from build123d import *

# Parameters (mm, degrees)
F0_R     = 4
F1_DEPTH = 15
F2_R     = 2.4
F3_DEPTH = 8
F4_SIZE  = 0.8
F5_R     = 11
F6_DEPTH = 5


with BuildPart() as f1:
    # F0 (on Top) → F1 (new body)
    with BuildSketch(Plane.XY):
        Circle(F0_R)
    extrude(amount=F1_DEPTH)

    # F2 (on face) → F3 (join)
    with BuildSketch(Plane.XY.offset(15)):
        Circle(F2_R)
    extrude(amount=F3_DEPTH)

    # F4
    f4_edges = [f1.edges().sort_by_distance(p)[0] for p in [
        (-2.4, 0, 23),
        (-4, 0, 0),
    ]]
    chamfer(f4_edges, length=F4_SIZE)

    # F5 (on Right) → F6 (cut, symmetric)
    with BuildSketch(Plane.YZ):
        with Locations((-13.5, 8)):
            Circle(F5_R)
        with Locations((13.5, 8)):
            Circle(F5_R)
    extrude(amount=F6_DEPTH, both=True, mode=Mode.SUBTRACT)


solid = f1.part
Model file for the job. Use its own axes, mm. Give positions to 0.01 mm unless a question says otherwise; leave off trailing zeros. Order: outer loops, then holes, each group sorted by start corner. A loop starts at its lowest first (then second) coordinate and runs counter-clockwise, first axis right, second up. Notation, with made-up numbers: (84, -2.75) - (103, -2.75) arc R31 ccw to (103, 34.25) - close; hole circle Ø3 at (-28.5, -34). An arc over 180 degrees is marked (long way). Write item = value, one per line. Start each with the question number.
1. Cut at A-A, the plane y = 0. List the corners of the cut face in (x, z).
2. Drop flat-ended pins along their axis: P1, Ø1, axis at x = 1.5, y = -2, coming from the +Z side; P2, Ø1.5, axis at x = 2, z = 7, coming from the -Y side. Give the stop position or say it passes through.
3. Cut at D-D, the plane z = 11.25. List the corners of the cut face in (x, y).
4. Cut at B-B, the plane x = 0. List the corners of the cut face in (y, z), and give its area (3 significant figures).
5. Cut at C-C, the plane z = 21. List the corners of the cut face in (x, y), and give its area (3 significant figures).
6. Probe line 1 along Z through (x, y) = (-2.5, -2); line 2 along X through (y, z) = (2.5, 6). List the from-to ranges inside material, lowest first.
7. Two-plate mould, pull along Z, no slides. Class faces 1 (the cylindrical face through (0, 2.5, 8.1)), 2 (the flat face through (2, -2, 15)), 3 (the cylindrical face through (0, -2.5, 7.9)), 4 (the cylindrical face through (1.29, 2.024, 18.55)): pulls with the +Z half, pulls with the -Z half, needs draft (parallel to the pull), parting line crosses it, or undercut.
Taken from the geometry:
q1.outline = (-4, 0.8) - (-3.2, 0) - (3.2, 0) - (4, 0.8) - (4, 15) - (2.4, 15) - (2.4, 22.2) - (1.6, 23) - (-1.6, 23) - (-2.4, 22.2) - (-2.4, 15) - (-4, 15) - close
q2.P1 = 22.6
q2.P2 = -2.64
q3.outline = (-2.66, -2.99) - (2.66, -2.99) arc R4 ccw to (2.66, 2.99) - (-2.66, 2.99) arc R4 ccw to start
q4.outline = (-4, 0.8) - (-3.2, 0) - (3.2, 0) - (4, 0.8) - (4, 2.45) arc R11 cw to (4, 13.55) - (4, 15) - (2.4, 15) - (2.4, 22.2) - (1.6, 23) - (-1.6, 23) - (-2.4, 22.2) - (-2.4, 15) - (-4, 15) - (-4, 13.55) arc R11 cw to (-4, 2.45) - close
q4.area = 135 mm²
q5.outline = circle Ø4.8 at (0, 0)
q5.area = 18.1 mm²
q6.line_1 = 0 to 15
q6.line_2 = -3.12 to 3.12
q7.face_1 = undercut
q7.face_2 = pulls with the +Z half
q7.face_3 = undercut
q7.face_4 = needs draft
